Autodesk Inventor part; units mm, degrees
ref_plane "YZ Plane" through (0, 0, 0) normal (1, 0, 0) x (0, 1, 0)
ref_plane "XZ Plane" through (0, 0, 0) normal (0, 1, 0) x (-1, 0, 0)
ref_plane "XY Plane" through (0, 0, 0) normal (0, 0, 1) x (1, 0, 0)
sketch "Sketch1" plane through (0, 0, 0) normal (0, 1, 0) x (-1, 0, 0)
  line L0 (-175, -169) -> (175, -169)
  line L1 (175, -169) -> (175, 169)
  line L2 (175, 169) -> (-175, 169)
  line L3 (-175, 169) -> (-175, -169)
  line L4 (-175, -169) -> (175, 169) construction
  line L5 (175, -169) -> (-175, 169) construction
  point P0 (0, 0)
  dimension "d0" = 338
  dimension "d1" = 350
extrude "Extrusion1" add sketch "Sketch1" along normal blind 12.7
sketch "Sketch2" plane through (0, 0, 0) normal (0, -1, 0) x (1, 0, 0)
  circle A0 centre (-97.564, 92.95) radius 12
  circle A1 centre (-97.564, -15.05) radius 12
  circle A2 centre (-97.564, -15.05) radius 12
  circle A3 centre (100.436, 92.95) radius 12
  circle A4 centre (100.436, -15.05) radius 12
  circle A5 centre (-125.564, 127) radius 6.73
  circle A6 centre (-125.564, 82.6) radius 6.73
  circle A7 centre (-125.564, -82.6) radius 6.73
  circle A8 centre (-125.564, -127) radius 6.73
  circle A9 centre (128.436, -127) radius 6.73
  circle A10 centre (128.436, -82.6) radius 6.73
  circle A11 centre (128.436, 82.6) radius 6.73
  circle A12 centre (128.436, 127) radius 6.73
  point P0 (0, 0)
extrude "Extrusion2" cut sketch "Sketch2" against normal blind 10
sketch "Sketch3" plane through (0, 0, 0) normal (0, -1, 0) x (1, 0, 0)
  circle A0 centre (-97.564, -15.05) radius 12
  circle A1 centre (-97.564, 92.95) radius 12
  circle A2 centre (100.436, -15.05) radius 12
  circle A3 centre (100.436, 92.95) radius 12
  point P0 (0, 0)
hole "Hole1" at (-97.564, 0, -15.05) at (-97.564, 0, 92.95) at (100.436, 0, -15.05) at (100.436, 0, 92.95) direction (0, 1, 0) diameter 26.211 depth 12.7
properties part number "PLACA BASE"
Geometry: final body of the model. Coordinates: model frame, mm. A direction names the side the tool comes from. Give positions to 0.01 mm unless a question says otherwise; leave off trailing zeros. Loops run counter-clockwise (first coordinate to the right, second up) from the corner with the lowest first, then second, coordinate; pieces in that order, holes last. Notation, with made-up numbers: (56, 0) - (98, 0) arc R18 cw to (98, 7) - close; hole circle Ø7 at (62, -30). An arc over 180 degrees is marked (long way). One line per question, with ' | ' between items. Start each with the question number.
(1) Contact query for flat-ended pins moving along their axis: pin 1 (4 mm diameter, centred on x = -126.5, z = 125, fed in from -Y); pin 2 (15.5 mm diameter, centred on x = 100.436, z = 92.95, fed in from +Y). Output: stop coordinate, or through.
(2) Section query B-B on z = 127. Return loops of the section in (x, y), then the cut area to 3 significant figures.
(3) Reachability of faces 1 (the cylindrical face through (-84.77, 6.44, -12.21)), 2 (the cylindrical face through (134.65, 4.93, 124.42)) from +Z, -Z, +X, -X, +Y, -Y: full face, straight path, thin tool, end or side. Return the list, or none.
(4) Pull-direction query (Z, two-part tool) for faces 3 (the flat face through (2, 12.7, 2)), 4 (the cylindrical face through (113.23, 6.44, -12.21)), 5 (the flat face through (-2, 6, 169)), 6 (the cylindrical face through (-119.35, 4.93, 124.42)); classes: released by +Z, released by -Z, zero draft, split by the parting line, or undercut.
(5) Section query C-C on y = 4.5. Count the separate pieces of the cut face and the enclosed holes in it, then the cut area to 3 significant figures.
(6) Section query A-A on z = -15.05. Return loops of the section in (x, y), then the cut area to 3 significant figures.
(7) Ray query, line 1 (X direction, y = 5, z = 92.95); line 2 (X direction, y = 4, z = -82.5); line 3 (Z direction, x = 97, y = 6). Return the intervals inside material, ascending. Write a range as from..to.
The answers:
1) pin 1: y = 10 | pin 2: through
2) outline: (-175, 0) - (-132.29, 0) - (-132.29, 10) - (-118.83, 10) - (-118.83, 0) - (121.71, 0) - (121.71, 10) - (135.17, 10) - (135.17, 0) - (175, 0) - (175, 12.7) - (-175, 12.7) - close | area: 4,180 mm2
3) face 1: +Y, -Y | face 2: -Y
4) face 3: zero draft | face 4: undercut | face 5: released by +Z | face 6: undercut
5) separate pieces: 1 | enclosed holes: 12 | area: 115,000 mm2
6) outline: (-175, 0) - (-110.67, 0) - (-110.67, 12.7) - (-175, 12.7) - close; (-84.46, 0) - (87.33, 0) - (87.33, 12.7) - (-84.46, 12.7) - close; (113.54, 0) - (175, 0) - (175, 12.7) - (113.54, 12.7) - close | area: 3,780 mm2
7) line 1: -175..-110.67, -84.46..87.33, 113.54..175 | line 2: -175..-132.29, -118.83..121.71, 135.17..175 | line 3: -169..-27.7, -2.4..80.3, 105.6..169
